from build123d import *

# Parameters (mm, degrees)
F0_W     = 576
F0_H     = 200
F1_DEPTH = 12
F3_D     = 5


with BuildPart() as f1:
    # F0 (on Right) → F1 (new body)
    with BuildSketch(Plane.YZ):
        with Locations((288, -100)):
            Rectangle(F0_W, F0_H)
    extrude(amount=F1_DEPTH)

    # F3 (through all)
    with Locations(Plane.XZ):
        with Locations((6, -20), (6, -180)):
            Hole(F3_D / 2)


solid = f1.part
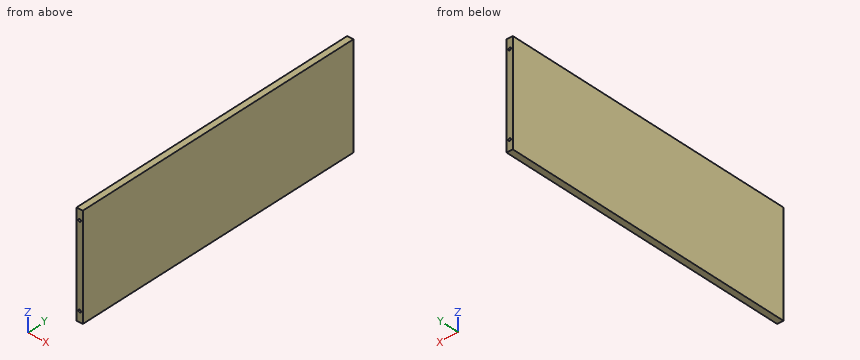
CAD build for the part. Positions are in the model's coordinates, mm. Round coordinates to 2 decimals unless told otherwise and drop trailing zeros. Write each loop counter-clockwise with the first axis right and the second up, starting at its lowest first coordinate (ties: lowest second). Pieces come first, ordered by that corner, then holes.
(1) Slice it at A-A, the plane x = 6. Write the cut outline in (y, z), and give its area (3 significant figures).
(2) Probe line 1 along Z through (x, y) = (6, 129); line 2 along X through (y, z) = (137, -180); line 3 along Z through (x, y) = (4.75, 381.5). List the from-to ranges inside material, lowest first.
(3) Drop a flat-ended pin along its axis: P1, Ø4.5, axis at x = 6, z = -180, coming from the -Y side. Give the stop position or say it passes through.
(4) Slice it at B-B, the plane y = 508. Write the cut outline in (x, z).
From the geometry:
1. outline: (0, -200) - (576, -200) - (576, -182.5) - (0, -182.5) - close; (0, -177.5) - (576, -177.5) - (576, -22.5) - (0, -22.5) - close; (0, -17.5) - (576, -17.5) - (576, 0) - (0, 0) - close
1. area: 109,000 mm2
2. line 1: z = -200 to -182.5, -177.5 to -22.5, -17.5 to 0
2. line 2: x = 0 to 3.5, 8.5 to 12
2. line 3: z = -200 to -182.17, -177.83 to -22.17, -17.83 to 0
3. P1: passes through
4. outline: (0, -200) - (12, -200) - (12, 0) - (0, 0) - close; hole circle Ø5 at (6, -180); hole circle Ø5 at (6, -20)
